from build123d import *

# Parameters (mm, degrees)
SCHIZZO1_W                   = 32.85
SCHIZZO1_H                   = 16.4
SCHIZZO1_W_2                 = 22.85
SCHIZZO1_H_2                 = 12.4
ESTRUSIONE_ESTRUSIONE1_DEPTH = 17.1
SCHIZZO2_W                   = 32.85
SCHIZZO2_H                   = 16.4
ESTRUSIONE_ESTRUSIONE2_DEPTH = 2
TAGLIO_ESTRUSIONE1_DEPTH     = 29.829683054
TAGLIO_ESTRUSIONE2_REACH     = 28.492
SCHIZZO16_W                  = 32.85
SCHIZZO16_H                  = 2
ESTRUSIONE_ESTRUSIONE3_DEPTH = 5


with BuildPart() as part:
    # Schizzo1 → Estrusione-Estrusione1 (new body)
    with BuildSketch(Plane.XY):
        Rectangle(SCHIZZO1_W, SCHIZZO1_H)
        Rectangle(SCHIZZO1_W_2, SCHIZZO1_H_2, mode=Mode.SUBTRACT)
    extrude(amount=ESTRUSIONE_ESTRUSIONE1_DEPTH)

    # Schizzo2 → Estrusione-Estrusione2 (add)
    with BuildSketch(Plane(origin=(0, 0, 0), x_dir=(-1, 0, 0), z_dir=(0, 0, -1))):
        Rectangle(SCHIZZO2_W, SCHIZZO2_H)
    extrude(amount=ESTRUSIONE_ESTRUSIONE2_DEPTH)

    # Schizzo8 → Foro per Vite M1-1 (revolve, cut)
    with BuildSketch(Plane(origin=(-13.925, 0, 17.1), x_dir=(0, -1, 0), z_dir=(1, 0, 0))):
        Polygon((0, 0), (0, 10.360516371), (0.6, 10), (0.6, 0), align=None)
    foro_per_vite_m1_1 = revolve(axis=Axis((-13.925, 0, 23.45), (0, 0, -1)), mode=Mode.SUBTRACT)

    # Specchia1: Foro per Vite M1-1 across plane
    add(foro_per_vite_m1_1.mirror(Plane(origin=(0, 0, 0), x_dir=(0, 0, 1), z_dir=(1, 0, 0))), mode=Mode.SUBTRACT)

    # Schizzo15 → Taglio-Estrusione1 (cut, through all)
    with BuildSketch(Plane.XZ.offset(8.2)):
        Polygon((16.425, -2), (1.425, -2), (16.425, 2.019237886), align=None)
    extrude(amount=-TAGLIO_ESTRUSIONE1_DEPTH, mode=Mode.SUBTRACT)

    # Schizzo16 → Taglio-Estrusione2 (cut, up to next)
    with BuildSketch(Plane.XY.offset(17.1), mode=Mode.PRIVATE) as taglio_estrusione2_sk1:
        with Locations((0, 7.2)):
            Rectangle(SCHIZZO16_W, SCHIZZO16_H)
    taglio_estrusione2_tool1 = extrude(taglio_estrusione2_sk1.sketch, amount=-TAGLIO_ESTRUSIONE2_REACH, mode=Mode.PRIVATE) & part.part
    add(taglio_estrusione2_tool1.solids().sort_by_distance((0, 7.2, 17.1))[0], mode=Mode.SUBTRACT)

    # Schizzo17 → Estrusione-Estrusione3 (add)
    with BuildSketch(Plane(origin=(0, 6.2, 0), x_dir=(1, 0, 0), z_dir=(0, 1, 0))):
        with BuildLine():
            Line((-16.425, -2.55), (-16.425, -12.55))
            ThreePointArc((-16.425, -12.55), (-21.425, -7.55), (-16.425, -2.55))
        make_face()
    estrusione_estrusione3 = extrude(amount=-ESTRUSIONE_ESTRUSIONE3_DEPTH)

    # Schizzo20 → Foro per Vite M2-1 (revolve, cut)
    with BuildSketch(Plane(origin=(-18.925, 1.2, 7.55), x_dir=(0, 0, -1), z_dir=(1, 0, 0))):
        Polygon((0, 0), (0, 10.721032743), (1.2, 10), (1.2, 0), align=None)
    foro_per_vite_m2_1 = revolve(axis=Axis((-18.925, -5.15, 7.55), (0, 1, 0)), mode=Mode.SUBTRACT)

    # Specchia2: Estrusione-Estrusione3, Foro per Vite M2-1 across plane
    add(estrusione_estrusione3.mirror(Plane(origin=(0, 0, 0), x_dir=(0, 0, 1), z_dir=(1, 0, 0))))
    add(foro_per_vite_m2_1.mirror(Plane(origin=(0, 0, 0), x_dir=(0, 0, 1), z_dir=(1, 0, 0))), mode=Mode.SUBTRACT)


solid = part.part
Check sheet for the modelled part. Datum: model origin and axes. Units: mm. A direction names the side the tool comes from. Give positions to 0.01 mm unless a question says otherwise; leave off trailing zeros. Loops run counter-clockwise (first coordinate to the right, second up) from the corner with the lowest first, then second, coordinate; pieces in that order, holes last. Notation, with made-up numbers: M 1,-18.5 L 9,-18.5 A22 ccw 9,20.5 Z; hole C 54,67.25 d5. An arc over 180 degrees is marked long. Use a Markdown table: item, result. Add a question column.
Q1. Tool access check on faces 1 (the flat face through (-11.425, 0, 8)), 2 (the flat face through (11.425, 0, 9)), 3 (the flat face through (-1, 0, 0)), 4 (the cylindrical face through (14.52, 0.08, 12.17)). Record the directions out of +Z, -Z, +X, -X, +Y, -Y that give a thin tool (end or side, any length) a straight path to the whole face; none if there is none.
Q2. Sectioned sample at B-B, the plane y = 2.25. Give the number of separate pieces and of enclosed holes in the cut face, then the cut area to 3 significant figures.
Q3. Sectioned sample at C-C, the plane z = 11.5. Record the cut outline in (x, y) (3 decimals).
Q4. Mould release check, pull along Y, two halves, no side actions. Record for faces 5 (the flat face through (15, 6.2, 9)), 6 (the flat face through (16.425, -3, 10)), 7 (the cylindrical face through (-14.52, 0.08, 12.17)): pulls with the +Y half, pulls with the -Y half, needs draft (parallel to the pull), parting line crosses it, or undercut.
Q5. Sectioned sample at D-D, the plane z = 7.55. Record the cut outline in (x, y) (3 decimals), then the cut area to 3 significant figures.
Q6. Go/stop test with flat-tipped pins: pin 1 (8 mm diameter, centred on y = -5.5, z = 7, fed in from -X) (3 decimals); pin 2 (4 mm diameter, centred on x = 18.925, z = 7.55, fed in from -Y); pin 3 (8 mm diameter, centred on y = -5.5, z = 0, fed in from +X) (3 decimals). Record where each tip stops, or that it passes through.
Q7. Sectioned sample at A-A, the plane y = -4.25. Record the cut outline in (x, z) (1 decimal), then the cut area to 3 significant figures.
Q8. Scan lines: line 1 along X through (y, z) = (0, 10.25) (3 decimals); line 2 along X through (y, z) = (-1.5, 5.5) (3 decimals); line 3 along X through (y, z) = (3.6, 7.55) (3 decimals). Record each from-to range of solid material in increasing order. Write a range as [from, to].
Verdict:
| question | item | result |
|---|---|---|
| 1 | face 1 | +Z, +Y |
| 1 | face 2 | +Z, -Z, +Y |
| 1 | face 3 | +Z, +X, +Y |
| 1 | face 4 | +Z |
| 2 | separate pieces | 2 |
| 2 | enclosed holes | 2 |
| 2 | area | 277 mm^2 |
| 3 | outline | M -19.491,1.2 L -16.425,1.2 L -16.425,-8.2 L 16.425,-8.2 L 16.425,1.2 L 19.491,1.2 L 19.491,6.2 L 11.425,6.2 L 11.425,-6.2 L -11.425,-6.2 L -11.425,6.2 L -19.491,6.2 Z; hole C -13.925,0 d1.2; hole C 13.925,0 d1.2 |
| 4 | face 5 | pulls with the +Y half |
| 4 | face 6 | needs draft |
| 4 | face 7 | undercut |
| 5 | outline | M -21.425,1.2 L -20.125,1.2 L -20.125,6.2 L -21.425,6.2 Z; M -17.725,1.2 L -16.425,1.2 L -16.425,-8.2 L 16.425,-8.2 L 16.425,1.2 L 17.725,1.2 L 17.725,6.2 L 11.425,6.2 L 11.425,-6.2 L -11.425,-6.2 L -11.425,6.2 L -17.725,6.2 Z; M 20.125,1.2 L 21.425,1.2 L 21.425,6.2 L 20.125,6.2 Z; hole C -13.925,0 d1.2; hole C 13.925,0 d1.2 |
| 5 | area | 213 mm^2 |
| 6 | pin 1 | x = -16.425 |
| 6 | pin 2 | y = 1.2 |
| 6 | pin 3 | x = 16.425 |
| 7 | outline | M -16.4,-2 L 1.4,-2 L 8.9,0 L -11.4,0 L -11.4,17.1 L -16.4,17.1 Z; M 11.4,0.7 L 16.4,2 L 16.4,17.1 L 11.4,17.1 Z |
| 7 | area | 207 mm^2 |
| 8 | line 1 | [-16.425, -14.525], [-13.325, -11.425], [11.425, 13.325], [14.525, 16.425] |
| 8 | line 2 | [-16.425, -11.425], [11.425, 16.425] |
| 8 | line 3 | [-21.425, -20.125], [-17.725, -11.425], [11.425, 17.725], [20.125, 21.425] |
